Design review of the part built by this model. Coordinates are the model's own, in mm. Face numbers are marked on the shaded views. A direction names the side the tool comes from. Give positions to 0.01 mm unless a question says otherwise; leave off trailing zeros. Loops run counter-clockwise (first coordinate to the right, second up) from the corner with the lowest first, then second, coordinate; pieces in that order, holes last.
from build123d import *

# Parameters (mm, degrees)
SKETCH1_W           = 25
SKETCH1_H           = 25
BOSS_EXTRUDE1_DEPTH = 22.5
SKETCH4_W           = 25
SKETCH4_H           = 25
BOSS_EXTRUDE2_DEPTH = 20
CUT_EXTRUDE2_DEPTH  = 42.5
CUT_EXTRUDE3_DEPTH  = 21
SKETCH6_R           = 2.25
CUT_EXTRUDE4_DEPTH  = 10
SKETCH8_W           = 45
SKETCH8_H           = 9.75
CUT_EXTRUDE5_DEPTH  = 50
SKETCH10_R          = 2.5
CUT_EXTRUDE7_DEPTH  = 10
CUT_EXTRUDE8_DEPTH  = 2.6


with BuildPart() as part:
    # Sketch1 → Boss-Extrude1 (new, symmetric)
    with BuildSketch(Plane(origin=(0, 0, 0), x_dir=(1, 0, 0), z_dir=(0, 1, 0))):
        Rectangle(SKETCH1_W, SKETCH1_H)
    extrude(amount=BOSS_EXTRUDE1_DEPTH, both=True)

    # Sketch4 → Boss-Extrude2 (add)
    with BuildSketch(Plane.ZY.offset(12.5)):
        with Locations((0, 10)):
            Rectangle(SKETCH4_W, SKETCH4_H)
    extrude(amount=BOSS_EXTRUDE2_DEPTH)

    # Sketch3 → Cut-Extrude2 (cut)
    with BuildSketch(Plane.XZ.offset(22.5)):
        Polygon((-2.75, 4.75), (-2.75, 10.25), (-10.25, 10.25), (-10.25, 2.75), (-4.75, 2.75), (-4.75, -2.75), (-10.25, -2.75), (-10.25, -10.25), (-2.75, -10.25), (-2.75, -4.75), (2.75, -4.75), (2.75, -10.25), (10.25, -10.25), (10.25, -2.75), (4.75, -2.75), (4.75, 2.75), (10.25, 2.75), (10.25, 10.25), (2.75, 10.25), (2.75, 4.75), align=None)
    extrude(amount=-CUT_EXTRUDE2_DEPTH, mode=Mode.SUBTRACT)

    # Sketch5 → Cut-Extrude3 (cut)
    with BuildSketch(Plane.ZY.offset(32.5)):
        Polygon((-10.5, 7.25), (-10.5, -0.5), (-2.75, -0.5), (-2.75, 5), (2.75, 5), (2.75, -0.5), (10.5, -0.5), (10.5, 7.25), (5, 7.25), (5, 12.75), (10.5, 12.75), (10.5, 20.5), (2.75, 20.5), (2.75, 15), (-2.75, 15), (-2.75, 20.5), (-10.5, 20.5), (-10.5, 12.75), (-5, 12.75), (-5, 7.25), align=None)
    extrude(amount=-CUT_EXTRUDE3_DEPTH, mode=Mode.SUBTRACT)

    # Sketch6 → Cut-Extrude4 (cut)
    with BuildSketch(Plane(origin=(0, 0, -12.5), x_dir=(-1, 0, 0), z_dir=(0, 0, -1))):
        with Locations((0, -12.5)):
            Circle(SKETCH6_R)
        with Locations((22.5, 10)):
            Circle(SKETCH6_R)
    extrude(amount=-CUT_EXTRUDE4_DEPTH, mode=Mode.SUBTRACT)

    # Sketch8 → Cut-Extrude5 (cut)
    with BuildSketch(Plane(origin=(0, 22.5, 0), x_dir=(1, 0, 0), z_dir=(0, 1, 0))):
        with Locations((-10, 7.625)):
            Rectangle(SKETCH8_W, SKETCH8_H)
    extrude(amount=-CUT_EXTRUDE5_DEPTH, mode=Mode.SUBTRACT)

    # Sketch10 → Cut-Extrude7 (cut)
    with BuildSketch(Plane.XY.offset(12.5)):
        with Locations((-27.5, 10)):
            Circle(SKETCH10_R)
        with Locations((0, -17.5)):
            Circle(SKETCH10_R)
    extrude(amount=-CUT_EXTRUDE7_DEPTH, mode=Mode.SUBTRACT)

    # Sketch11 → Cut-Extrude8 (cut)
    with BuildSketch(Plane(origin=(0, 0, 4.75), x_dir=(-1, 0, 0), z_dir=(0, 0, -1))):
        Polygon((2.222626661, -13.550219745), (-2.309296709, -13.600258721), (-4.53192337, -17.550038976), (-2.222626661, -21.449780255), (2.309296709, -21.399741279), (4.53192337, -17.449961024), align=None)
        Polygon((31.438967259, 12.241733763), (27.528085243, 14.532112593), (23.589117983, 12.29037883), (23.561032741, 7.758266237), (27.471914757, 5.467887407), (31.410882017, 7.70962117), align=None)
    extrude(amount=-CUT_EXTRUDE8_DEPTH, mode=Mode.SUBTRACT)


solid = part.part
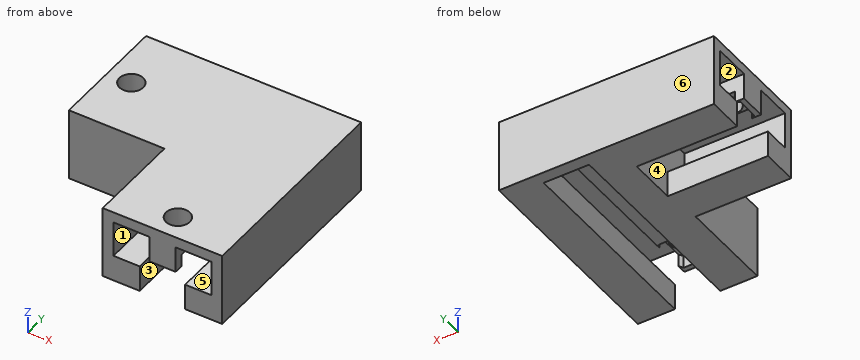
Q1. Take a section at A-A (x = -27.5). Give the boundary of the cut face in (y, z).
Results:
outline: (-2.5, -2.75) - (5, -2.75) - (5, 2.75) - (-0.5, 2.75) - (-0.5, 10.5) - (7.25, 10.5) - (7.25, 7.35) - (7.5, 7.35) - (7.5, 12.5) - (-2.5, 12.5) - close; (12.5, 7.35) - (12.75, 7.35) - (12.75, 10.5) - (20.5, 10.5) - (20.5, 2.75) - (15, 2.75) - (15, -2.75) - (22.5, -2.75) - (22.5, 12.5) - (12.5, 12.5) - close
Q2. Insertion check: pin 1 (4.5 mm diameter, centred on x = -21, z = 8, fed in from -Y); pin 2 (3 mm diameter, centred on x = 0, y = -17.5, fed in from -Z); pin 3 (5 mm diameter, centred on x = -16, y = 10, fed in from -Z); pin 4 (2 mm diameter, centred on y = 15.5, z = 8.5, fed in from -X). Each pin has a flat end and moves straight along its axis. Give the tip position at first contact, or say it passes through.
Results:
pin 1: stops at y = -2.5
pin 2: passes through
pin 3: stops at z = 5
pin 4: stops at x = -11.5
Q3. Draft analysis for pull direction Y (two halves, no side actions). For the marked faces 4, 5 and 6, state which applies: pulls with the +Y half, pulls with the -Y half, needs draft (parallel to the pull), parting line crosses it, or undercut.
Results:
face 4: undercut
face 5: needs draft
face 6: pulls with the +Y half
Q4. Take a section at C-C (z = 4). Give the boundary of the cut face in (x, y).
Results:
outline: (-32.5, -2.5) - (-12.5, -2.5) - (-12.5, -22.5) - (-10.25, -22.5) - (-10.25, 20) - (10.25, 20) - (10.25, -22.5) - (12.5, -22.5) - (12.5, 22.5) - (-32.5, 22.5) - (-32.5, 20.5) - (-11.5, 20.5) - (-11.5, -0.5) - (-32.5, -0.5) - close
Q5. Wall thickness on line 1 (X direction, y = -10, z = 9.25); line 2 (Y direction, x = -17, z = 5.75); line 3 (Y direction, x = -27.5, z = 10.45): over which ranges is each line inside the solid? List them lowest first.
Results:
line 1: x = -12.5 to -10.25, -2.75 to 2.75, 10.25 to 12.5
line 2: y = -2.5 to -0.5, 7.25 to 12.75, 20.5 to 22.5
line 3: y = -2.5 to -0.5, 7.25 to 7.5, 12.5 to 12.75, 20.5 to 22.5
Q6. Take a section at D-D (x = -3.5). Give the boundary of the cut face in (y, z), plus the area to 3 significant figures.
Results:
outline: (-22.5, 10.25) - (20, 10.25) - (20, -2.75) - (22.5, -2.75) - (22.5, 12.5) - (-22.5, 12.5) - close
area: 134 mm2
Q7. Take a section at B-B (y = -17.5). Give the boundary of the cut face in (x, z).
Results:
outline: (-12.5, -2.75) - (-4.75, -2.75) - (-4.75, 2.75) - (-10.25, 2.75) - (-10.25, 10.25) - (-2.75, 10.25) - (-2.75, 7.35) - (-2.5, 7.35) - (-2.5, 12.5) - (-12.5, 12.5) - close; (2.5, 7.35) - (2.75, 7.35) - (2.75, 10.25) - (10.25, 10.25) - (10.25, 2.75) - (4.75, 2.75) - (4.75, -2.75) - (12.5, -2.75) - (12.5, 12.5) - (2.5, 12.5) - close
Q8. Tool access review of the marked faces 1, 2 and 3: name each direction out of +Z, -Z, +X, -X, +Y, -Y from which nothing blocks a thin tool from reaching the whole face with its end or side.
Results:
face 1: -Y
face 2: -X
face 3: -Z, -Y
